Read the model definition and answer for the solid it produces. Units are mm, in the model's axes. A direction names the side the tool comes from. Coordinates: 2 decimals unless noted, no trailing zeros. Loops run counter-clockwise (first coordinate to the right, second up) from the corner with the lowest first, then second, coordinate; pieces in that order, holes last.
from build123d import *

# Parameters (mm, degrees)
PAD_DEPTH    = 10
FILLET_R     = 1
CHAMFER_SIZE = 0.4


with BuildPart() as part:
    # Sketch → Pad (new body)
    with BuildSketch(Plane.XY):
        with BuildLine():
            Line((-18.5, 55), (-22.5, 55))
            Line((-22.5, 55), (-22.5, 74))
            Line((-22.5, 74), (22.5, 74))
            Line((22.5, 74), (22.5, 6))
            ThreePointArc((22.5, 6), (24.5, 4), (26.5, 6))
            Line((26.5, 6), (26.5, 30))
            ThreePointArc((30.5, 30), (28.5, 32), (26.5, 30))
            Line((30.5, 30), (30.5, 0))
            Line((30.5, 0), (18.5, 0))
            Line((18.5, 0), (18.5, 70))
            Line((18.5, 70), (-18.5, 70))
            Line((-18.5, 70), (-18.5, 55))
        make_face()
    extrude(amount=PAD_DEPTH)

    # Fillet
    fillet_edges = [part.edges().sort_by_distance(p)[0] for p in [
        (18.5, 70, 5),
        (-18.5, 55, 5),
        (-22.5, 55, 5),
        (-22.5, 74, 5),
        (22.5, 74, 5),
        (18.5, 0, 5),
        (30.5, 0, 5),
        (-18.5, 70, 5),
    ]]
    fillet(fillet_edges, radius=FILLET_R)

    # Chamfer
    chamfer_edges = [part.edges().sort_by_distance(p)[0] for p in [
        (30.5, 15.5, 10),
        (30.207107, 0.292893, 10),
        (28.5, 32, 10),
        (24.5, 0, 10),
        (26.5, 18, 10),
        (18.792893, 0.292893, 10),
        (24.5, 4, 10),
        (18.5, 35, 10),
        (22.5, 39.5, 10),
        (18.207107, 69.707107, 10),
        (22.207107, 73.707107, 10),
        (0, 70, 10),
        (0, 74, 10),
        (-18.207107, 69.707107, 10),
        (-22.207107, 73.707107, 10),
        (-18.5, 62.5, 10),
        (-22.5, 64.5, 10),
        (-18.792893, 55.292893, 10),
        (-22.207107, 55.292893, 10),
        (-20.5, 55, 10),
        (30.5, 15.5, 0),
        (30.207107, 0.292893, 0),
        (28.5, 32, 0),
        (24.5, 0, 0),
        (26.5, 18, 0),
        (18.792893, 0.292893, 0),
        (24.5, 4, 0),
        (18.5, 35, 0),
        (22.5, 39.5, 0),
        (18.207107, 69.707107, 0),
        (22.207107, 73.707107, 0),
        (0, 70, 0),
        (0, 74, 0),
        (-18.207107, 69.707107, 0),
        (-22.207107, 73.707107, 0),
        (-18.5, 62.5, 0),
        (-22.5, 64.5, 0),
        (-18.792893, 55.292893, 0),
        (-22.207107, 55.292893, 0),
        (-20.5, 55, 0),
    ]]
    chamfer(chamfer_edges, length=CHAMFER_SIZE)


solid = part.part
Item 1: Given pin 1 (4.5 mm diameter, centred on y = 42, z = 7, fed in from +X); pin 2 (3 mm diameter, centred on x = -8.5, z = 3, fed in from -Y); pin 3 (3 mm diameter, centred on y = 32, z = 2.5, fed in from -X), each flat-ended and moving along its own axis, determine where each tip first touches the part or whether it passes through.
Numbers:
pin 1: stops at x = 22.5
pin 2: stops at y = 70
pin 3: stops at x = 18.5
Item 2: A cutting plane is placed at A-A on y = 16. Determine the outline of the cut face in (x, z), then the cut area to 3 significant figures.
Numbers:
outline: (18.5, 0.4) - (18.9, 0) - (22.1, 0) - (22.5, 0.4) - (22.5, 9.6) - (22.1, 10) - (18.9, 10) - (18.5, 9.6) - close; (26.5, 0.4) - (26.9, 0) - (30.1, 0) - (30.5, 0.4) - (30.5, 9.6) - (30.1, 10) - (26.9, 10) - (26.5, 9.6) - close
area: 79.4 mm2
Item 3: Find the intervals of material crossed by line 1 along X through (y, z) = (23.5, 0.5); line 2 along X through (y, z) = (68.5, 2.25); line 3 along X through (y, z) = (42.5, 2), in increasing order.
Numbers:
line 1: x = 18.5 to 22.5, 26.5 to 30.5
line 2: x = -22.5 to -18.5, 18.5 to 22.5
line 3: x = 18.5 to 22.5
Item 4: Which of the six approach directions +Z, -Z, +X, -X, +Y, -Y give full straight-line access (tool end or side, diameter ignored) to faces 5 (the face through (22.5, 40, 5)), 6 (the face through (18.5, 35, 5)), 7 (the face through (-20, 55, 5)), 8 (the face through (18.32, 69.81, 9.75))?
Numbers:
face 5: +Z, -Z, +Y
face 6: +Z, -Z, -Y
face 7: +Z, -Z, -X, -Y
face 8: +Z, -Y
Item 5: A cutting plane is placed at D-D on y = 48.5. Determine the outline of the cut face in (x, z), then the cut area to 3 significant figures.
Numbers:
outline: (18.5, 0.4) - (18.9, 0) - (22.1, 0) - (22.5, 0.4) - (22.5, 9.6) - (22.1, 10) - (18.9, 10) - (18.5, 9.6) - close
area: 39.7 mm2
Item 6: A cutting plane is placed at B-B on z = 6. Determine the outline of the cut face in (x, y), then the cut area to 3 significant figures.
Numbers:
outline: (-22.5, 56) arc R1 ccw to (-21.5, 55) - (-19.5, 55) arc R1 ccw to (-18.5, 56) - (-18.5, 69) arc R1 cw to (-17.5, 70) - (17.5, 70) arc R1 cw to (18.5, 69) - (18.5, 1) arc R1 ccw to (19.5, 0) - (29.5, 0) arc R1 ccw to (30.5, 1) - (30.5, 30) arc R2 ccw to (26.5, 30) - (26.5, 6) arc R2 cw to (22.5, 6) - (22.5, 73) arc R1 ccw to (21.5, 74) - (-21.5, 74) arc R1 ccw to (-22.5, 73) - close
area: 663 mm2
Item 7: Determine the mould class of faces 1 (the face through (-22.5, 64, 5)), 2 (the face through (20, 43, 0)), 3 (the face through (18.32, 69.81, 0.25)), 4 (the face through (24.45, 3.89, 0.29)) for opening direction X: released by +X, released by -X, zero draft, split by the parting line, or undercut.
Numbers:
face 1: released by -X
face 2: zero draft
face 3: undercut
face 4: undercut
Item 8: A cutting plane is placed at C-C on x = 28.5. Determine the outline of the cut face in (y, z).
Numbers:
outline: (0, 0.4) - (0.4, 0) - (31.6, 0) - (32, 0.4) - (32, 9.6) - (31.6, 10) - (0.4, 10) - (0, 9.6) - close
